Geometry: final body of the model. Coordinates: model frame, mm. A direction names the side the tool comes from. Round coordinates to 2 decimals unless told otherwise and drop trailing zeros. Order: outer loops, then holes, each group sorted by start corner. A loop starts at its lowest first (then second) coordinate and runs counter-clockwise, first axis right, second up. Notation, with made-up numbers: M 3.25,69.25 L 33.25,69.25 A14 ccw 33.25,94.25 Z; hole C 18.5,12 d4. An arc over 180 degrees is marked long. Put each result on its own line as item: value. Start each with the question number.
1) Section C-C, the plane z = 1.3. Count the separate pieces of the cut face and the enclosed holes in it, then the cut area to 3 significant figures.
2) First-contact query: P1, Ø1.8, axis at x = -18.09, y = 77.05, coming from the -Z side; P2, Ø0.9, axis at x = -13, z = 1.5, coming from the -Y side; P3, Ø5, axis at x = 10, y = -47, coming from the -Z side; P4, Ø1, axis at y = 25, z = 2, coming from the -X side. Flat tips, straight axial feed; report the tip coordinate or a pass-through.
3) Draft query along X for faces 1 (the flat face through (54.62, -54.274, 1.521)), 2 (the flat face through (49.55, -74.3, 1.52)), 3 (the cylindrical face through (0.853, 99.996, 1.479)), 4 (the flat face through (-49.55, 74.3, 1.52)). Return one class per face: pulls with the +X half, pulls with the -X half, needs draft (parallel to the pull), parting line crosses it, or undercut.
4) Section B-B, the plane x = 0. Return loops of the section in (y, z).
5) Section D-D, the plane x = 75.5. Return loops of the section in (y, z).
6) Material intervals for probe 1 along X at (y, z) = (-48.5, 1.2); probe 2 along X at (y, z) = (55, 1.9); probe 3 along X at (y, z) = (46, 0.6), sorted ascending. Write a range as [from, to].
7) Access query for faces 5 (the flat face through (54.274, 54.62, 1.521)), 6 (the flat face through (49.765, 74.514, 1.521)), 7 (the flat face through (74.3, 49.55, 1.52)), 8 (the cylindrical face through (84.7, 53.16, 1.48)). Directions: +Z, -Z, +X, -X, +Y, -Y. A direction counts if a zero-diameter tool reaches every point of the face in a straight line with its end or side. Return the directions, or none.
8) Section A-A, the plane y = 0. Return loops of the section in (x, z).
from build123d import *

# Parameters (mm, degrees)
CROQUIS1_R              = 100
SALIENTE_EXTRUIR1_DEPTH = 3
CROQUIS3_R              = 110
CORTAR_EXTRUIR1_DEPTH   = 3
REDONDEO1_R             = 10
CROQUIS4_R              = 1.5
CROQUIS4_R_2            = 12.5
CORTAR_EXTRUIR2_DEPTH   = 142.453172607
CROQUIS6_R              = 1.5
CROQUIS6_W              = 7.95
CROQUIS6_H              = 6
CROQUIS6_W_2            = 6
CROQUIS6_H_2            = 7.95
CORTAR_EXTRUIR3_DEPTH   = 10
CROQUIS8_R              = 1.5
CORTAR_EXTRUIR5_DEPTH   = 142.453172607


with BuildPart() as part:
    # Croquis1 → Saliente-Extruir1 (new body)
    with BuildSketch(Plane.XY):
        Circle(CROQUIS1_R)
    extrude(amount=SALIENTE_EXTRUIR1_DEPTH)

    # Croquis3 → Cortar-Extruir1 (cut)
    with BuildSketch(Plane.XY.offset(3)):
        with Locations((190, 0)):
            Circle(CROQUIS3_R)
    extrude(amount=-CORTAR_EXTRUIR1_DEPTH, mode=Mode.SUBTRACT)

    # Redondeo1
    redondeo1_edges = [part.edges().sort_by_distance(p)[0] for p in [
        (89.473684211, -44.659375654, 1.5),
        (89.473684211, 44.659375654, 1.5),
    ]]
    fillet(redondeo1_edges, radius=REDONDEO1_R)

    # Croquis4 → Cortar-Extruir2 (cut, through all)
    with BuildSketch(Plane.XY.offset(3)):
        with Locations((-65.01846853, -38.219121523)):
            Circle(CROQUIS4_R)
        with Locations((-49.462119344, -22.662772337)):
            Circle(CROQUIS4_R)
        with Locations((-22.662772337, -49.462119344)):
            Circle(CROQUIS4_R)
        with Locations((-38.219121523, -65.01846853)):
            Circle(CROQUIS4_R)
        with Locations((-22.662772337, 49.462119344)):
            Circle(CROQUIS4_R)
        with Locations((-38.219121523, 65.01846853)):
            Circle(CROQUIS4_R)
        with Locations((-49.462119344, 22.662772337)):
            Circle(CROQUIS4_R)
        with Locations((-65.01846853, 38.219121523)):
            Circle(CROQUIS4_R)
        with Locations((49.462119344, 22.662772337)):
            Circle(CROQUIS4_R)
        with Locations((65.01846853, 38.219121523)):
            Circle(CROQUIS4_R)
        with Locations((22.662772337, 49.462119344)):
            Circle(CROQUIS4_R)
        with Locations((38.219121523, 65.01846853)):
            Circle(CROQUIS4_R)
        with Locations((22.662772337, -49.462119344)):
            Circle(CROQUIS4_R)
        with Locations((38.219121523, -65.01846853)):
            Circle(CROQUIS4_R)
        with Locations((49.462119344, -22.662772337)):
            Circle(CROQUIS4_R)
        with Locations((65.01846853, -38.219121523)):
            Circle(CROQUIS4_R)
        Circle(CROQUIS4_R_2)
        Polygon((-58.336309448, -83.085046789), (-83.085046789, -58.336309448), (-66.821590822, -42.072853481), (-42.072853481, -66.821590822), align=None)
        Polygon((-66.821590822, 42.072853481), (-42.072853481, 66.821590822), (-58.336309448, 83.085046789), (-83.085046789, 58.336309448), align=None)
        Polygon((42.072853481, 66.821590822), (66.821590822, 42.072853481), (83.085046789, 58.336309448), (58.336309448, 83.085046789), align=None)
        Polygon((66.821590822, -42.072853481), (42.072853481, -66.821590822), (58.336309448, -83.085046789), (83.085046789, -58.336309448), align=None)
    extrude(amount=-CORTAR_EXTRUIR2_DEPTH, mode=Mode.SUBTRACT)

    # Croquis6 → Cortar-Extruir3 (cut)
    with BuildSketch(Plane.XY.offset(3)):
        with Locations((70, 18.09)):
            Circle(CROQUIS6_R)
        with Locations((62.05, 18.09)):
            Circle(CROQUIS6_R)
        with Locations((62.05, -18.09)):
            Circle(CROQUIS6_R)
        with Locations((-18.09, 85)):
            Circle(CROQUIS6_R)
        with Locations((-18.09, 77.05)):
            Circle(CROQUIS6_R)
        with Locations((18.09, 85)):
            Circle(CROQUIS6_R)
        with Locations((18.09, 77.05)):
            Circle(CROQUIS6_R)
        with Locations((70, -18.09)):
            Circle(CROQUIS6_R)
        with Locations((18.09, -77.05)):
            Circle(CROQUIS6_R)
        with Locations((18.09, -85)):
            Circle(CROQUIS6_R)
        with Locations((-18.09, -85)):
            Circle(CROQUIS6_R)
        with Locations((-18.09, -77.05)):
            Circle(CROQUIS6_R)
        with Locations((-77.05, -18.09)):
            Circle(CROQUIS6_R)
        with Locations((-85, -18.09)):
            Circle(CROQUIS6_R)
        with Locations((-85, 18.09)):
            Circle(CROQUIS6_R)
        with Locations((-77.05, 18.09)):
            Circle(CROQUIS6_R)
        with Locations((66.025, -13.09)):
            Rectangle(CROQUIS6_W, CROQUIS6_H)
        with Locations((13.09, 81.025)):
            Rectangle(CROQUIS6_W_2, CROQUIS6_H_2)
        with Locations((-13.09, -81.025)):
            Rectangle(CROQUIS6_W_2, CROQUIS6_H_2)
        with Locations((-81.025, 13.09)):
            Rectangle(CROQUIS6_W, CROQUIS6_H)
    extrude(amount=-CORTAR_EXTRUIR3_DEPTH, mode=Mode.SUBTRACT)

    # Croquis8 → Cortar-Extruir5 (cut, through all)
    with BuildSketch(Plane.XY.offset(3)):
        with Locations((-55.578593001, 39.173715678)):
            Circle(CROQUIS8_R)
        with Locations((-39.173715678, 55.578593001)):
            Circle(CROQUIS8_R)
        with Locations((-20.718228689, 4.313351365)):
            Circle(CROQUIS8_R)
        with Locations((-4.313351365, 20.718228689)):
            Circle(CROQUIS8_R)
        with Locations((39.173715678, 55.578593001)):
            Circle(CROQUIS8_R)
        with Locations((55.578593001, 39.173715678)):
            Circle(CROQUIS8_R)
        with Locations((20.718228689, 4.313351365)):
            Circle(CROQUIS8_R)
        with Locations((4.313351365, 20.718228689)):
            Circle(CROQUIS8_R)
        with Locations((55.578593001, -39.173715678)):
            Circle(CROQUIS8_R)
        with Locations((39.173715678, -55.578593001)):
            Circle(CROQUIS8_R)
        with Locations((4.313351365, -20.718228689)):
            Circle(CROQUIS8_R)
        with Locations((20.718228689, -4.313351365)):
            Circle(CROQUIS8_R)
        with Locations((-39.173715678, -55.578593001)):
            Circle(CROQUIS8_R)
        with Locations((-55.578593001, -39.173715678)):
            Circle(CROQUIS8_R)
        with Locations((-20.718228689, -4.313351365)):
            Circle(CROQUIS8_R)
        with Locations((-4.313351365, -20.718228689)):
            Circle(CROQUIS8_R)
    extrude(amount=-CORTAR_EXTRUIR5_DEPTH, mode=Mode.SUBTRACT)


solid = part.part
Result sheet:
1. separate pieces: 1
1. enclosed holes: 53
1. area: 26,000 mm2
2. P1: passes through
2. P2: stops at y = -99.21
2. P3: stops at z = 0
2. P4: stops at x = -96.95
3. face 1: undercut
3. face 2: pulls with the +X half
3. face 3: parting line crosses it
3. face 4: pulls with the -X half
4. outline: M -100,0 L -12.5,0 L -12.5,3 L -100,3 Z; M 12.5,0 L 100,0 L 100,3 L 12.5,3 Z
5. outline: M -50.75,0 L 50.75,0 L 50.75,3 L -50.75,3 Z
6. probe 1: x = [-87.45, -73.25], [-60.39, -23.81], [-21.51, 21.51], [23.81, 60.39], [73.25, 87.43]
6. probe 2: x = [-83.52, -79.75], [-53.89, -40.56], [-37.79, 37.79], [40.56, 53.89], [79.75, 83.52]
6. probe 3: x = [-88.79, -70.75], [-62.89, 62.89], [70.75, 88.25]
7. face 5: +Z, -Z
7. face 6: +Z, -Z, +X
7. face 7: +Z, -Z, +Y
7. face 8: +Z, -Z, +X, +Y
8. outline: M -100,0 L -12.5,0 L -12.5,3 L -100,3 Z; M 12.5,0 L 80,0 L 80,3 L 12.5,3 Z
